from build123d import *

# Parameters (mm, degrees)
F0_W      = 12.7
F0_H      = 114.3
F1_DEPTH  = 25.4
F2_W      = 19.05
F2_H      = 12.7
F3_DEPTH  = 12.701
F4_R      = 6.34999
F5_R      = 3.175
F6_DEPTH  = 25.401
F8_DEPTH  = 6.35
F10_DEPTH = 6.35


# Not quite as in the source:
# - a fillet or chamfer is up to 0.001 mm smaller than in the source, because OpenCascade refuses the exact size


with BuildPart() as f1:
    # F0 (on Top) → F1 (new body)
    with BuildSketch(Plane.XY):
        with Locations((6.35, 57.15)):
            Rectangle(F0_W, F0_H)
    extrude(amount=F1_DEPTH)

    # F2 (on face) → F3 (cut, through all)
    with BuildSketch(Plane.YZ.offset(12.7)):
        with Locations((9.525, 12.7)):
            Rectangle(F2_W, F2_H)
    extrude(amount=-F3_DEPTH, mode=Mode.SUBTRACT)

    # F4 (radius 6.35 in the source; OpenCascade refuses exactly that, so slightly less here)
    f4_edges = [f1.edges().sort_by_distance(p)[0] for p in [
        (12.7, 0, 22.225),
        (12.7, 0, 3.175),
        (0, 0, 3.175),
        (0, 0, 22.225),
    ]]
    fillet(f4_edges, radius=F4_R)

    # F5 (on face) → F6 (cut, through all)
    with BuildSketch(Plane.XY.offset(25.4)):
        with Locations((6.35, 9.525)):
            Circle(F5_R)
    extrude(amount=-F6_DEPTH, mode=Mode.SUBTRACT)

    # F7 (on face) → F8 (join, through all)
    with BuildSketch(Plane.XY.offset(25.4)):
        with BuildLine():
            Line((0, 6.35), (0, 20.5235226281))
            ThreePointArc((0, 20.5235226281), (6.35, -3.175), (12.7, 20.5235226281))
            Line((12.7, 20.5235226281), (12.7, 6.35))
            ThreePointArc((12.7, 6.35), (6.35, 0), (0, 6.35))
        make_face()
    extrude(amount=-F8_DEPTH)

    # F9 (on face) → F10 (join, through all)
    with BuildSketch(Plane.XY.offset(25.4)):
        with BuildLine():
            ThreePointArc((21.59, 12.6358519733), (21.7481397779, 12.663985398), (21.9075, 12.6840851128))
            ThreePointArc((21.9075, 12.6840851128), (21.9058819686, 12.6920429708), (21.9042598667, 12.7))
            Line((21.9042598667, 12.7), (21.59, 12.6358519733))
        make_face()
        with BuildLine():
            ThreePointArc((21.9075, 6.3659148872), (25.4, 9.525), (21.9075, 12.6840851128))
            ThreePointArc((21.9075, 12.6840851128), (21.7481397779, 12.663985398), (21.59, 12.6358519733))
            Line((21.59, 12.6358519733), (18.7934078933, 12.065))
            ThreePointArc((18.7934078933, 12.065), (19.05, 9.525), (18.7934078933, 6.985))
            Line((18.7934078933, 6.985), (21.59, 6.4141480267))
            ThreePointArc((21.59, 6.4141480267), (21.7481397779, 6.386014602), (21.9075, 6.3659148872))
        make_face()
        with BuildLine():
            ThreePointArc((21.9042598667, 6.35), (21.9058819686, 6.3579570292), (21.9075, 6.3659148872))
            ThreePointArc((21.9075, 6.3659148872), (21.7481397779, 6.386014602), (21.59, 6.4141480267))
            Line((21.59, 6.4141480267), (21.9042598667, 6.35))
        make_face()
    extrude(amount=-F10_DEPTH)


solid = f1.part
Can you work these out from the model? Positions are in its coordinate system, mm. A direction names the side the tool comes from. Round coordinates to 2 decimals unless told otherwise and drop trailing zeros. Write each loop counter-clockwise with the first axis right and the second up, starting at its lowest first coordinate (ties: lowest second). Pieces come first, ordered by that corner, then holes. Notation, with made-up numbers: (52.5, -18.5) - (67.5, -18.5) arc R16 ccw to (67.5, -7.5) - close; hole circle Ø3 at (7, 40). An arc over 180 degrees is marked (long way). Write each question's results on one line, items separated by ' | '. Start each with the question number.
1) Suppose I cut it at C-C (x = 8). List the corners of the cut face in (y, z) for me.
2) We'd pull the mould along X, two halves only. Please class faces 5 (the flat face through (0, 60, 13)), 6 (the flat face through (6, 58, 0)), 7 (the flat face through (12.7, 60, 13)), 8 (the cylindrical face through (4.01, 11.67, 22.27)): released by +X, released by -X, zero draft, split by the parting line, or undercut.
3) Suppose I cut it at B-B (y = 16). List the corners of the cut face in (x, z) for me, and give its area (3 significant figures).
4) Please list where these lines run through material, in increasing order: line 1 (Y direction, x = 6.35, z = 4.5); line 2 (X direction, y = 30.5, z = 2.5); line 3 (Z direction, x = 15.5, y = 5.5).
5) For pin 1 Ø3 at (y, z) = (11.5, 17.5) entering from -X; pin 2 Ø7.5 at (y, z) = (35.5, 7.5) entering from -X; pin 3 Ø8 at (y, z) = (77, 11) entering from +X; pin 4 Ø12 at (x, z) = (12, 16.5) entering from -Y, each with a flat end and sliding along its axis, tell me the tip position at first contact or that it passes through.
6) Which directions (+Z, -Z, +X, -X, +Y, -Y) give clear straight access to the entire face, cutting with the end or side of a thin tool? Please do faces 1 (the cylindrical face through (1.81, 1.91, 3.22)), 2 (the flat face through (4, 12, 6.35)), 3 (the cylindrical face through (10.79, 1.81, 3.22)), 4 (the flat face through (6, 43, 25.4)).
7) Suppose I cut it at D-D (y = 106). List the corners of the cut face in (x, z) for me.
Here are the results:
1) outline: (-3.07, 19.05) - (6.81, 19.05) - (6.81, 25.4) - (-3.07, 25.4) - close; (0.22, 0) - (6.81, 0) - (6.81, 6.35) - (0.22, 6.35) - close; (12.24, 0) - (114.3, 0) - (114.3, 25.4) - (12.24, 25.4) - (12.24, 19.05) - (19.05, 19.05) - (19.05, 6.35) - (12.24, 6.35) - close
2) face 5: released by -X | face 6: zero draft | face 7: released by +X | face 8: undercut
3) outline: (-4.58, 19.05) - (17.28, 19.05) - (17.28, 25.4) - (-4.58, 25.4) - close; (0, 0) - (12.7, 0) - (12.7, 6.35) - (0, 6.35) - close | area: 219 mm2
4) line 1: y = 0 to 6.35, 12.7 to 114.3 | line 2: x = 0 to 12.7 | line 3: z = 19.05 to 25.4
5) pin 1: passes through | pin 2: stops at x = 0 | pin 3: stops at x = 12.7 | pin 4: stops at y = -3.17
6) face 1: -Z, -X, -Y | face 2: +X, -X, -Y | face 3: -Z, +X, -Y | face 4: +Z, +X, -X, +Y, -Y
7) outline: (0, 0) - (12.7, 0) - (12.7, 25.4) - (0, 25.4) - close
